For this review, take the finished solid that the model builds, in its own axes (mm). Face numbers are marked on the shaded views. A direction names the side the tool comes from. Coordinates: 2 decimals unless noted, no trailing zeros. Write each loop counter-clockwise with the first axis right and the second up, starting at its lowest first coordinate (ties: lowest second). Pieces come first, ordered by that corner, then holes.
1) To check wall thickness, follow line 1 along X through (y, z) = (16, 0) (1 decimal); line 2 along X through (y, z) = (47, 0) (1 decimal); line 3 along Z through (x, y) = (1, 46) (3 decimals). State the ranges of each line that lie inside material, in increasing order.
2) For the marked faces 1, 2, 3, 4 and 5, list the 3-axis set-ups (+Z, -Z, +X, -X, +Y, -Y) from which the entire face can be reached by the end or side of a thin tool; tool diameter is ignored.
3) Mouldability with a two-part tool opening along X and no side actions: class the marked faces 6, 7 and 8 as pulls with the +X half, pulls with the -X half, needs draft (parallel to the pull), parting line crosses it, or undercut.
4) We need section B-B on z = 9. Write out the cut boundary in (x, y) (3 decimals).
5) Insertion check: P1, Ø3, axis at x = 19.5, y = 44, coming from the -Z side; P2, Ø14.5, axis at x = 3, y = 26.5, coming from the -Z side; P3, Ø4, axis at x = 0.5, y = 59, coming from the -Z side (3 decimals); P4, Ø4, axis at x = -11, z = -1.5, coming from the -Y side. Each pin has a flat end and moves straight along its axis. Give the tip position at first contact, or say it passes through.
6) We need section D-D on x = -12.5. Write out the cut boundary in (y, z) (3 decimals), then the cut area to 3 significant figures.
7) We need section A-A on y = 51. Write out the cut boundary in (x, z) (1 decimal).
from build123d import *

# Parameters (mm, degrees)
SKETCH1_R           = 11.1125
BOSS_EXTRUDE1_DEPTH = 79.375
BOSS_EXTRUDE2_REACH = 92.43
SKETCH2_R           = 15.875


with BuildPart() as part:
    # Sketch1 → Boss-Extrude1 (new body)
    with BuildSketch(Plane(origin=(0, 0, 0), x_dir=(1, 0, 0), z_dir=(0, 1, 0))):
        Polygon((6.575640303, -15.875), (15.875, -6.575640303), (15.875, 6.575640303), (6.575640303, 15.875), (-6.575640303, 15.875), (-15.875, 6.575640303), (-15.875, -6.575640303), (-6.575640303, -15.875), align=None)
        with Locations(Location((0, 0, 0), (0, 0, 90))):
            Circle(SKETCH1_R, mode=Mode.SUBTRACT)
    extrude(amount=BOSS_EXTRUDE1_DEPTH)

    # Sketch2 → Boss-Extrude2 (add, up to next)
    with BuildSketch(Plane(origin=(14.760854057, 0, -14.760854057), x_dir=(-0.7071067811865476, 0, -0.7071067811865475), z_dir=(0.7071067811865475, 0, -0.7071067811865476)), mode=Mode.PRIVATE) as boss_extrude2_sk1:
        with Locations((0, 39.634677984)):
            Circle(SKETCH2_R)
    boss_extrude2_tool1 = extrude(boss_extrude2_sk1.sketch, amount=-BOSS_EXTRUDE2_REACH, mode=Mode.PRIVATE) - part.part
    add(boss_extrude2_tool1.solids().sort_by_distance((14.760854, 39.634678, -14.760854))[0])


solid = part.part
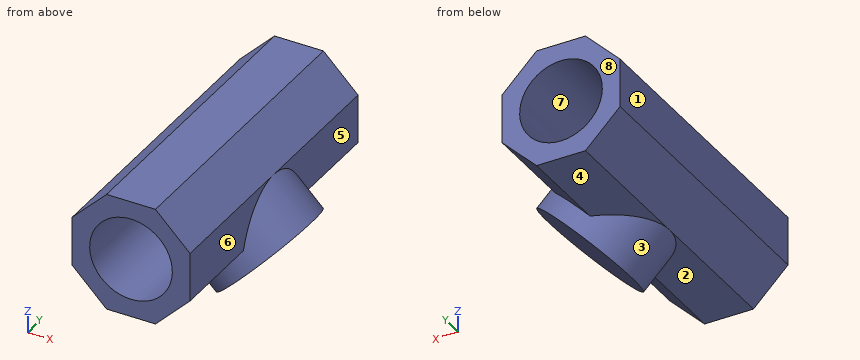
Result:
1. line 1: x = -15.9 to -11.1, 11.1 to 15.9
1. line 2: x = -15.9 to -11.1, 11.1 to 19.9
1. line 3: z = -21.567 to -11.067, 11.067 to 15.875
2. face 1: +Z, -Z, -X, +Y, -Y
2. face 2: -Z, -X, -Y
2. face 3: none
2. face 4: -Z, -X, +Y
2. face 5: +Z, +X, +Y
3. face 6: pulls with the +X half
3. face 7: undercut
3. face 8: needs draft
4. outline: (-13.451, 0) - (-6.518, 0) - (-6.518, 79.375) - (-13.451, 79.375) - close; (6.518, 0) - (13.451, 0) - (13.451, 79.375) - (6.518, 79.375) - close
5. P1: stops at z = -11.52
5. P2: stops at z = -25.15
5. P3: stops at z = -15.875
5. P4: stops at y = 0
6. outline: (0, -9.951) - (79.375, -9.951) - (79.375, 9.951) - (0, 9.951) - close
6. area: 1,580 mm2
7. outline: (-15.9, -6.6) - (-6.6, -15.9) - (0.2, -15.9) - (6.9, -22.6) - (22.6, -6.9) - (15.9, -0.2) - (15.9, 6.6) - (6.6, 15.9) - (-6.6, 15.9) - (-15.9, 6.6) - close; hole circle Ø22.2 at (0, 0)
